Autodesk Inventor part; units mm, degrees
ref_plane "YZ Plane" through (0, 0, 0) normal (1, 0, 0) x (0, 1, 0)
ref_plane "XZ Plane" through (0, 0, 0) normal (0, 1, 0) x (-1, 0, 0)
ref_plane "XY Plane" through (0, 0, 0) normal (0, 0, 1) x (1, 0, 0)
sketch "Sketch1" plane through (0, 0, 0) normal (0, 0, 1) x (1, 0, 0)
  line L0 (-33.8048, 23.6808) -> (143.9952, 23.6808)
  line L1 (143.9952, 23.6808) -> (143.9952, 4.6308)
  line L2 (143.9952, 4.6308) -> (-33.8048, 4.6308)
  line L3 (-33.8048, 4.6308) -> (-33.8048, 23.6808)
  point P0 (0, 0)
  dimension "d0" = 177.8
  dimension "d1" = 19.05
extrude "Extrusion1" add sketch "Sketch1" along normal blind 50.8
sketch "Sketch2" plane through (0, 0, 50.8) normal (0, 0, 1) x (1, 0, 0)
  circle A0 centre (136.3752, 14.1558) radius 6.35
  line L0 (143.9952, 4.6308) -> (143.9952, 23.6808)
  line L1 (-33.8048, 4.6308) -> (143.9952, 4.6308)
  point P0 (0, 0)
  dimension "d4" = 12.7
  dimension "d5" = 7.62
  dimension "d6" = 9.525
extrude "Extrusion2" cut sketch "Sketch2" against normal blind 50.8
sketch "Sketch3" plane through (-33.8048, 23.6808, 0) normal (0, 1, 0) x (1, 0, 0)
  line L0 (0, 0) -> (0, -50.8)
  line L1 (0, -31.75) -> (19.05, -31.75)
  line L2 (19.05, -31.75) -> (19.05, -19.05)
  line L3 (19.05, -19.05) -> (0, -19.05)
  line L4 (0, -19.05) -> (0, -31.75)
  line L5 (177.8, 0) -> (0, 0)
  point P0 (33.8048, 0)
  point P1 (0, -19.05)
  dimension "d9" = 19.05
  dimension "d10" = 12.7
  dimension "d11" = 19.05
extrude "Extrusion3" cut sketch "Sketch3" against normal blind 50.8
sketch "Sketch4" plane through (-33.8048, 23.6808, 19.05) normal (0, 0, 1) x (1, 0, 0)
  circle A0 centre (6.35, -9.525) radius 3.175
  line L0 (19.05, 0) -> (19.05, -19.05)
  line L1 (0, -19.05) -> (177.8, -19.05)
  point P0 (33.8048, -23.6808)
  dimension "d14" = 6.35
  dimension "d15" = 12.7
  dimension "d16" = 9.525
extrude "Extrusion4" cut sketch "Sketch4" along normal mid plane 127
properties part number "Ramp Base"
Source: CAD feature listing. Evaluate the final solid. Frame: model axes, mm. A direction names the side the tool comes from. Coordinates: 2 decimals unless noted, no trailing zeros. Loops run counter-clockwise (first coordinate to the right, second up) from the corner with the lowest first, then second, coordinate; pieces in that order, holes last. Notation, with made-up numbers: (76.25, 67.25) - (131.25, 67.25) arc R25 ccw to (131.25, 82.25) - close; hole circle Ø5 at (-8.75, -23). An arc over 180 degrees is marked (long way). One line per item, written item: value. Start each with the question number.
1. Contact query for a flat-ended pin moving along its axis: P1, Ø1, axis at y = 21.5, z = 26, coming from the -X side. Output: stop coordinate, or through.
2. Section B-B (y = 22). Return the cut outline in (x, z), and give its area (3 significant figures).
3. Ray query, L1, parallel to X at y = 14, z = 2; L2, parallel to X at y = 11.5, z = 32.5; L3, parallel to X at y = 21.75, z = 26.5. Return the intervals inside material, ascending.
4. Section A-A (x = -19.5). Return the cut outline in (y, z), and give its area (3 significant figures).
5. Section D-D (z = 24). Return the cut outline in (x, y), and give its area (3 significant figures).
6. Set-up query: faces 1 (the flat face through (-14.755, 14, 25)), 2 (the flat face through (54, 23.681, 25)). Return all of +Z, -Z, +X, -X, +Y, -Y with unobstructed straight access to the full face (end or side cutting, diameter ignored); none if empty.
7. Mould query, pull axis X, two halves, no side actions, for faces 3 (the flat face through (54, 14, 50.8)), 4 (the cylindrical face through (-24.426, 13.202, 41.142)), 5 (the flat face through (-33.805, 14, 41)), 6 (the cylindrical face through (130.03, 14.43, 25.76)). Classes: pulls with the +X half, pulls with the -X half, needs draft (parallel to the pull), parting line crosses it, or undercut.
8. Section C-C (z = 10). Return the cut outline in (x, y) (3 decimals), and give its area (3 significant figures).
Verdict:
1. P1: stops at x = -14.75
2. outline: (-33.8, 0) - (144, 0) - (144, 50.8) - (-33.8, 50.8) - (-33.8, 31.75) - (-14.75, 31.75) - (-14.75, 19.05) - (-33.8, 19.05) - close
2. area: 8,790 mm2
3. L1: x = -33.8 to -30.63, -24.28 to 130.03, 142.72 to 144
3. L2: x = -33.8 to -29.19, -25.71 to 130.61, 142.14 to 144
3. L3: x = -14.75 to 144
4. outline: (4.63, 0) - (23.68, 0) - (23.68, 19.05) - (4.63, 19.05) - close; (4.63, 31.75) - (23.68, 31.75) - (23.68, 50.8) - (4.63, 50.8) - close
4. area: 726 mm2
5. outline: (-14.75, 4.63) - (144, 4.63) - (144, 23.68) - (-14.75, 23.68) - close; hole circle Ø12.7 at (136.38, 14.16)
5. area: 2,900 mm2
6. face 1: -X, +Y, -Y
6. face 2: +Z, -Z, +X, -X, +Y
7. face 3: needs draft
7. face 4: undercut
7. face 5: pulls with the -X half
7. face 6: undercut
8. outline: (-33.805, 4.631) - (143.995, 4.631) - (143.995, 23.681) - (-33.805, 23.681) - close; hole circle Ø6.35 at (-27.455, 14.156); hole circle Ø12.7 at (136.375, 14.156)
8. area: 3,230 mm2
